Verification items for the finished model (mm, model axes). A direction names the side the tool comes from. Give positions to 0.01 mm unless a question says otherwise; leave off trailing zeros. Order: outer loops, then holes, each group sorted by start corner. A loop starts at its lowest first (then second) coordinate and runs counter-clockwise, first axis right, second up. Notation, with made-up numbers: (57, 85.5) - (88, 85.5) arc R21 cw to (88, 117.5) - close; hole circle Ø1 at (-7, 27). An arc over 180 degrees is marked (long way). Answer as a JSON object with one key per item and string values.
```python
from build123d import *

# Parameters (mm, degrees)
SKETCH_1_W               = 12
SKETCH_1_H               = 4.8
SKETCH_1_R               = 0.95
EXTRUDE_1_DEPTH          = 5
EXTRUDE_1_2_DEPTH        = 5
SKETCH_2_W               = 15.7
SKETCH_2_H               = 32.6
EXTRUDE_2_DEPTH          = 3
SKETCH_3_W               = 3
SKETCH_3_H               = 32.6
EXTRUDE_3_DEPTH          = 10
SKETCH_6_R               = 3
CUT_EXTRUDE_1_DEPTH      = 38.872549426
SKETCH_7_W               = 10.7
SKETCH_7_H               = 4.8
EXTRUDE_5_DEPTH          = 12
SKETCH_9_W               = 4.4
SKETCH_9_H               = 5.2
CUT_EXTRUDE_2_DEPTH      = 2.5
SKETCH_10_W              = 4.4
SKETCH_10_H              = 1
CUT_EXTRUDE_3_DEPTH      = 2.5
CUT_EXTRUDE_4_DEPTH      = 12.5
CUT_EXTRUDE_4_DEPTH_BACK = 12.5
SKETCH_11_W              = 1
SKETCH_11_H              = 2.3
SKETCH_12_W              = 10.7
SKETCH_12_H              = 2.4
CUT_EXTRUDE_5_DEPTH      = 12
CUT_EXTRUDE_6_DEPTH      = 12
SKETCH_14_R              = 3
EXTRUDE_6_DEPTH          = 3
CUT_EXTRUDE_7_DEPTH      = 23


with BuildPart() as part:
    # Sketch 1 → Extrude 1 (new body)
    with BuildSketch(Plane.XY):
        Rectangle(SKETCH_1_W, SKETCH_1_H)
        Circle(SKETCH_1_R, mode=Mode.SUBTRACT)
    extrude(amount=EXTRUDE_1_DEPTH)



with BuildPart() as body_2:
    # Sketch 1 → Extrude 1 2 (new body)
    with BuildSketch(Plane.XY):
        with Locations((0, -27.8)):
            Rectangle(SKETCH_1_W, SKETCH_1_H)
        with Locations((0, -27.8)):
            Circle(SKETCH_1_R, mode=Mode.SUBTRACT)
    extrude(amount=EXTRUDE_1_2_DEPTH)


with BuildPart() as part_1:
    add(part.part)

    add(body_2.part)  # Extrude 2 merges body 2
    # Sketch 2 → Extrude 2 (add)
    with BuildSketch(Plane(origin=(6, 0, 0), x_dir=(0, 0, -1), z_dir=(1, 0, 0))):
        with Locations((2.85, -13.9)):
            Rectangle(SKETCH_2_W, SKETCH_2_H)
    extrude(amount=EXTRUDE_2_DEPTH)

    # Sketch 3 → Extrude 3 (add)
    with BuildSketch(Plane(origin=(9, 0, 0), x_dir=(0, 0, -1), z_dir=(1, 0, 0))):
        with Locations((9.2, -13.9)):
            Rectangle(SKETCH_3_W, SKETCH_3_H)
    extrude(amount=EXTRUDE_3_DEPTH)

    # Sketch 6 → Cut-Extrude 1 (cut, through all)
    with BuildSketch(Plane.XY.offset(-7.7)):
        with Locations((14, -7.6169052)):
            Circle(SKETCH_6_R)
    extrude(amount=-CUT_EXTRUDE_1_DEPTH, mode=Mode.SUBTRACT)

    # Sketch 7 → Extrude 5 (add)
    with BuildSketch(Plane.ZY.offset(-6)):
        with Locations((-5.35, 0)):
            Rectangle(SKETCH_7_W, SKETCH_7_H)
    extrude(amount=EXTRUDE_5_DEPTH)

    # Sketch 9 → Cut-Extrude 2 (cut)
    with BuildSketch(Plane(origin=(0, 2.4, 0), x_dir=(1, 0, 0), z_dir=(0, 1, 0))):
        with Locations((0, 3.734554069)):
            Rectangle(SKETCH_9_W, SKETCH_9_H)
    extrude(amount=-CUT_EXTRUDE_2_DEPTH, mode=Mode.SUBTRACT)

    # Sketch 10 → Cut-Extrude 3 (cut)
    with BuildSketch(Plane(origin=(0, -0.1, 0), x_dir=(1, 0, 0), z_dir=(0, 1, 0))):
        with Locations((0, 5.834554069)):
            Rectangle(SKETCH_10_W, SKETCH_10_H)
        with Locations((0, 1.634554069)):
            Rectangle(SKETCH_10_W, SKETCH_10_H)
    extrude(amount=-CUT_EXTRUDE_3_DEPTH, mode=Mode.SUBTRACT)

    # Sketch 11 → Cut-Extrude 4 (cut, two sides: drawn at the far end of the back side and taken through both)
    with BuildSketch(Plane.ZY.offset(-2.2).offset(-CUT_EXTRUDE_4_DEPTH_BACK)):
        with Locations((-1.634554069, -1.25)):
            Rectangle(SKETCH_11_W, SKETCH_11_H)
        with Locations((-5.834554069, -1.25)):
            Rectangle(SKETCH_11_W, SKETCH_11_H)
    extrude(amount=CUT_EXTRUDE_4_DEPTH + CUT_EXTRUDE_4_DEPTH_BACK, mode=Mode.SUBTRACT)

    # Sketch 12 → Cut-Extrude 5 (cut)
    with BuildSketch(Plane.ZY.offset(6)):
        with Locations((-5.35, -1.2)):
            Rectangle(SKETCH_12_W, SKETCH_12_H)
    extrude(amount=-CUT_EXTRUDE_5_DEPTH, mode=Mode.SUBTRACT)

    # Sketch 13 → Cut-Extrude 6 (cut)
    with BuildSketch(Plane.XY.offset(-7.7)):
        with BuildLine():
            Line((14, -2.6169052), (9, -2.6169052))
            Line((9, -2.6169052), (9, 2.4))
            Line((9, 2.4), (19, 2.4))
            Line((19, 2.4), (19, -7.6169052))
            ThreePointArc((19, -7.6169052), (17.535533906, -4.081371294), (14, -2.6169052))
        make_face()
    extrude(amount=-CUT_EXTRUDE_6_DEPTH, mode=Mode.SUBTRACT)

    # Sketch 14 → Extrude 6 (add)
    with BuildSketch(Plane(origin=(0, 0, -10.7), x_dir=(-1, 0, 0), z_dir=(0, 0, -1))):
        with BuildLine():
            Line((-19, -7.6169052), (-19, -30.2))
            Line((-19, -30.2), (-6, -30.2))
            Line((-6, -30.2), (-6, 0))
            Line((-6, 0), (6, 0))
            Line((6, 0), (6, 2.4))
            Line((6, 2.4), (-9, 2.4))
            Line((-9, 2.4), (-9, -2.6169052))
            Line((-9, -2.6169052), (-14, -2.6169052))
            ThreePointArc((-14, -2.6169052), (-17.535533906, -4.081371294), (-19, -7.6169052))
        make_face()
        with Locations(Location((-14, -7.6169052, 0), (0, 0, 180))):
            Circle(SKETCH_14_R, mode=Mode.SUBTRACT)
    extrude(amount=EXTRUDE_6_DEPTH)

    # Sketch 15 → Cut-Extrude 7 (cut)
    with BuildSketch(Plane.XY.offset(5)):
        with BuildLine():
            Line((9, -2.6), (9, 2.4))
            Line((9, 2.4), (4, 2.4))
            ThreePointArc((4, 2.4), (7.535533906, 0.935533906), (9, -2.6))
        make_face()
    extrude(amount=-CUT_EXTRUDE_7_DEPTH, mode=Mode.SUBTRACT)


solid = part_1.part
```
(1) Release check for a two-part mould opening along X. For faces 4 (the cylindrical face through (-0.95, 0.04, 2.46)), 5 (the flat face through (8, -1, -2.135)), 6 (the flat face through (-6, -28, 2)) record: pulls with the +X half, pulls with the -X half, needs draft (parallel to the pull), parting line crosses it, or undercut.
Computed values:
{"face 4": "undercut", "face 5": "needs draft", "face 6": "pulls with the -X half"}
(2) Access from +Z, -Z, +X, -X, +Y, -Y to the whole of each face (thin tool, end or side, straight path). Record for faces 1 (the flat face through (0, 1, -6.335)), 2 (the flat face through (7.2, -0.1, -1.6)), 3 (the flat face through (14, -17, -7.7)).
Computed values:
{"face 1": "+Y, -Y", "face 2": "+X, -X", "face 3": "+Z, +X, +Y, -Y"}
(3) Section check C-C (z = 4.25). Record the cut outline in (x, y), then the cut area to 3 significant figures.
Computed values:
{"outline": "(-6, -30.2) - (9, -30.2) - (9, -2.6) arc R5 ccw to (4, 2.4) - (-6, 2.4) - (-6, -2.4) - (6, -2.4) - (6, -25.4) - (-6, -25.4) - close; hole circle Ø1.9 at (0, -27.8); hole circle Ø1.9 at (0, 0)", "area": "202 mm²"}
(4) Material ranges on line 1 along Y through (x, z) = (0, 1.3); line 2 along Y through (x, z) = (10.75, -8); line 3 along Y through (x, z) = (-1.25, -10), recorded low to high. Write a range as [from, to].
Computed values:
{"line 1": "y = [-30.2, -28.75], [-26.85, -25.4], [-2.4, -0.95], [0.95, 2.4]", "line 2": "y = [-30.2, -2.62]", "line 3": "y = [0, 2.4]"}
(5) Section check D-D (x = 4.5). Record the cut outline in (y, z), then the cut area to 3 significant figures.
Computed values:
{"outline": "(-30.2, 0) - (-25.4, 0) - (-25.4, 5) - (-30.2, 5) - close; (-2.4, 0) - (0, 0) - (0, -13.7) - (2.37, -13.7) - (2.37, 5) - (-2.4, 5) - close", "area": "80.4 mm²"}
(6) Section check B-B (y = -27.8). Record the cut outline in (x, z), then the cut area to 3 significant figures.
Computed values:
{"outline": "(-6, 0) - (-0.95, 0) - (-0.95, 5) - (-6, 5) - close; (0.95, 0) - (6, 0) - (6, -13.7) - (19, -13.7) - (19, -7.7) - (9, -7.7) - (9, 5) - (0.95, 5) - close", "area": "167 mm²"}
(7) Section check A-A (x = 0). Record the cut outline in (y, z).
Computed values:
{"outline": "(-30.2, 0) - (-28.75, 0) - (-28.75, 5) - (-30.2, 5) - close; (-26.85, 0) - (-25.4, 0) - (-25.4, 5) - (-26.85, 5) - close; (-2.4, 0) - (-0.95, 0) - (-0.95, 5) - (-2.4, 5) - close; (0, -13.7) - (2.4, -13.7) - (2.4, -6.33) - (0, -6.33) - close; (0, -1.13) - (2.4, -1.13) - (2.4, 5) - (0.95, 5) - (0.95, 0) - (0, 0) - close"}
(8) Gauge pin test, flat ends, axial feed: pin 1 Ø0.5 at (x, z) = (7.5, -1.5) entering from +Y; pin 2 Ø4 at (y, z) = (-25.5, -3) entering from +X; pin 3 Ø3 at (x, y) = (16.5, -18.5) entering from +Z; pin 4 Ø3 at (x, z) = (16.5, -4.5) entering from -Y. Record the tip position at first contact, or that the pin passes through.
Computed values:
{"pin 1": "stops at y = 1.2", "pin 2": "stops at x = 9", "pin 3": "stops at z = -7.7", "pin 4": "passes through"}
